Check sheet for the modelled part. Datum: model origin and axes. Units: mm. A direction names the side the tool comes from. Coordinates: 2 decimals unless noted, no trailing zeros. Loops run counter-clockwise (first coordinate to the right, second up) from the corner with the lowest first, then second, coordinate; pieces in that order, holes last. Notation, with made-up numbers: M 84,-17 L 125,-17 A26 cw 125,-3 Z; hole C 18.5,-2.75 d2. An arc over 180 degrees is marked long. Answer in a Markdown table with one row per item. Add a question column.
```python
from build123d import *

# Parameters (mm, degrees)
BOSS_EXTRUDE1_DEPTH = 331.978
FILLET1_R           = 2.54
FILLET2_R           = 2.54
SKETCH2_R           = 12.7
CUT_EXTRUDE1_DEPTH  = 335.699723609


with BuildPart() as part:
    # Sketch1 → Boss-Extrude1 (new body)
    with BuildSketch(Plane.XY):
        Polygon((0, 0), (38.1, 0), (38.1, -19.05), (33.02, -19.05), (33.02, -4.572), (-33.02, -4.572), (-33.02, -19.05), (-38.1, -19.05), (-38.1, 0), align=None)
    extrude(amount=BOSS_EXTRUDE1_DEPTH)

    # Fillet1
    fillet1_edges = [part.edges().sort_by_distance(p)[0] for p in [
        (-33.02, -4.572, 165.989),
    ]]
    fillet(fillet1_edges, radius=FILLET1_R)

    # Fillet2
    fillet2_edges = [part.edges().sort_by_distance(p)[0] for p in [
        (33.02, -4.572, 165.989),
    ]]
    fillet(fillet2_edges, radius=FILLET2_R)

    # Sketch2 → Cut-Extrude1 (cut, through all)
    with BuildSketch(Plane(origin=(0, 0, 0), x_dir=(1, 0, 0), z_dir=(0, 1, 0))):
        with Locations(Location((0, -316.738, 0), (0, 0, 270))):
            Circle(SKETCH2_R)
    extrude(amount=-CUT_EXTRUDE1_DEPTH, mode=Mode.SUBTRACT)


solid = part.part
```
Q1. Cross-section at A-A (x = 0). Record the cut outline in (y, z).
Q2. Mould release check, pull along Z, two halves, no side actions. Record for faces 1 (the face through (1, -3, 331.978)), 2 (the face through (-33.02, -13, 164)), 3 (the face through (0.56, -2.25, 304.05)), 4 (the face through (1, -3, 0)): released by +Z, released by -Z, zero draft, split by the parting line, or undercut.
Q3. Cross-section at C-C (z = 179). Record the cut outline in (x, y).
Q4. Thickness scan on L1, parallel to X at y = -15, z = 134; L2, parallel to Y at x = -4.5, z = 196; L3, parallel to Z at x = -2.5, y = -0.75. Record the ranges inside material, lowest first.
Q5. Access from +Z, -Z, +X, -X, +Y, -Y to the whole of each face (thin tool, end or side, straight path). Record for faces 5 (the face through (1, 0, 164)), 6 (the face through (0, -4.572, 164)).
Q6. Cross-section at B-B (y = -14). Record the cut outline in (x, z), plus the area to 3 significant figures.
Q7. Go/stop test with flat-tipped pins: pin 1 (8 mm diameter, centred on x = -18, y = -12.5, fed in from -Z); pin 2 (3 mm diameter, centred on x = 17.5, z = 210.5, fed in from -Y). Record where each tip stops, or that it passes through.
Q8. Cross-section at D-D (x = 19). Record the cut outline in (y, z), plus the area to 3 significant figures.
Answer key:
| question | item | result |
|---|---|---|
| 1 | outline | M -4.57,0 L 0,0 L 0,304.04 L -4.57,304.04 Z; M -4.57,329.44 L 0,329.44 L 0,331.98 L -4.57,331.98 Z |
| 2 | face 1 | released by +Z |
| 2 | face 2 | zero draft |
| 2 | face 3 | undercut |
| 2 | face 4 | released by -Z |
| 3 | outline | M -38.1,-19.05 L -33.02,-19.05 L -33.02,-7.11 A2.54 cw -30.48,-4.57 L 30.48,-4.57 A2.54 cw 33.02,-7.11 L 33.02,-19.05 L 38.1,-19.05 L 38.1,0 L -38.1,0 Z |
| 4 | L1 | -38.1 to -33.02, 33.02 to 38.1 |
| 4 | L2 | -4.57 to 0 |
| 4 | L3 | 0 to 304.29, 329.19 to 331.98 |
| 5 | face 5 | +Z, -Z, +X, -X, +Y |
| 5 | face 6 | +Z, -Z, -Y |
| 6 | outline | M -38.1,0 L -33.02,0 L -33.02,331.98 L -38.1,331.98 Z; M 33.02,0 L 38.1,0 L 38.1,331.98 L 33.02,331.98 Z |
| 6 | area | 3,370 mm^2 |
| 7 | pin 1 | through |
| 7 | pin 2 | y = -4.57 |
| 8 | outline | M -4.57,0 L 0,0 L 0,331.98 L -4.57,331.98 Z |
| 8 | area | 1,520 mm^2 |
